Here's how the part is built. I have some questions about the finished solid (model axes, mm). Face numbers are marked on the shaded views. A direction names the side the tool comes from. Give positions to 0.01 mm unless a question says otherwise; leave off trailing zeros. Write each loop counter-clockwise with the first axis right and the second up, starting at its lowest first coordinate (ties: lowest second). Pieces come first, ordered by that corner, then holes. Notation, with made-up numbers: (23, 27.25) -> (81, 27.25) arc R11 cw to (81, 43.25) -> close; hole circle Ø1 at (86, 6.5). An arc over 180 degrees is marked (long way). Return JSON: item names as keys, results as strings.
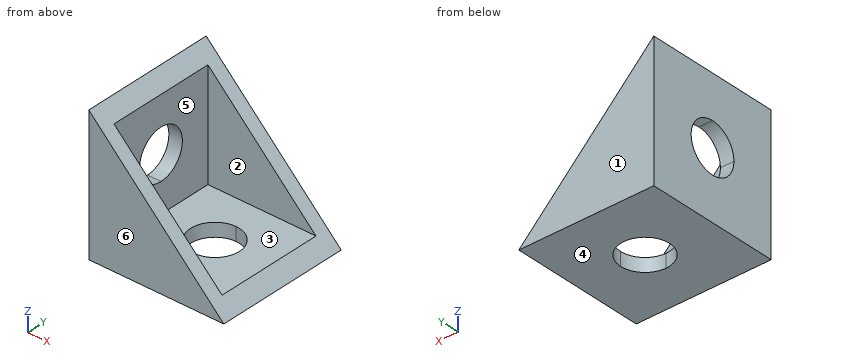
from build123d import *

# Parameters (mm, degrees)
F0_W     = 12.7
F0_H     = 12.7
F1_DEPTH = 12.7
F3_DEPTH = 25.4
F4_T     = -1.27
F7_DEPTH = 25.4
F8_DEPTH = 25.4


with BuildPart() as f1:
    # F0 (on Top) → F1 (new body)
    with BuildSketch(Plane.XY):
        with Locations((4.3248645961, 3.1129373469)):
            Rectangle(F0_W, F0_H)
    extrude(amount=F1_DEPTH)

    # F2 (on face) → F3 (cut)
    with BuildSketch(Plane.XZ.offset(3.2370626531)):
        Polygon((10.6748645961, 12.7), (-2.0251354039, 12.7), (10.6748645961, 0), align=None)
    extrude(amount=-F3_DEPTH, mode=Mode.SUBTRACT)

    # F4
    f4_openings = [f1.faces().sort_by_distance(p)[0] for p in [
        (4.324865, 3.112937, 6.35),
    ]]
    offset(amount=F4_T, openings=f4_openings)

    # F6 (on face) → F7 (cut)
    with BuildSketch(Plane(origin=(-2.0251354039, 0, 0), x_dir=(0, -1, 0), z_dir=(-1, 0, 0))):
        with BuildLine():
            ThreePointArc((-0.8015373469, 6.35), (-1.4785307329, 7.984406614), (-3.1129373469, 8.6614))
            Line((-3.1129373469, 8.6614), (-3.1129373469, 4.0386))
            ThreePointArc((-3.1129373469, 4.0386), (-1.4785307329, 4.715593386), (-0.8015373469, 6.35))
        make_face()
        with BuildLine():
            Line((-3.1129373469, 4.0386), (-3.1129373469, 8.6614))
            ThreePointArc((-3.1129373469, 8.6614), (-5.4243373469, 6.35), (-3.1129373469, 4.0386))
        make_face()
    extrude(amount=-F7_DEPTH, mode=Mode.SUBTRACT)

    # F5 (on face) → F8 (cut)
    with BuildSketch(Plane(origin=(0, 0, 0), x_dir=(1, 0, 0), z_dir=(0, 0, -1))):
        with BuildLine():
            ThreePointArc((6.6108645961, -3.1129373469), (5.9413106979, -1.4964912451), (4.3248645961, -0.8269373469))
            Line((4.3248645961, -0.8269373469), (4.3248645961, -5.3989373469))
            ThreePointArc((4.3248645961, -5.3989373469), (5.9413106979, -4.7293834487), (6.6108645961, -3.1129373469))
        make_face()
        with BuildLine():
            Line((4.3248645961, -5.3989373469), (4.3248645961, -0.8269373469))
            ThreePointArc((4.3248645961, -0.8269373469), (2.0388645961, -3.1129373469), (4.3248645961, -5.3989373469))
        make_face()
    extrude(amount=-F8_DEPTH, mode=Mode.SUBTRACT)


solid = f1.part
1. If we mould it in two halves opening along Y, with no side actions, what happens to the marked faces 3, 4, 5 and 6? For each: released by +Y, released by -Y, zero draft, split by the parting line, or undercut.
Taken from the geometry:
{"face 3": "undercut", "face 4": "zero draft", "face 5": "undercut", "face 6": "released by -Y"}
2. Suppose I cut it at A-A, the plane y = 1.75. List the corners of the cut face in (x, z) for me, and give its area (3 significant figures).
Taken from the geometry:
{"outline": "(-2.03, 0) -> (2.49, 0) -> (2.49, 1.27) -> (-0.76, 1.27) -> (-0.76, 4.48) -> (-2.03, 4.48) -> close; (-2.03, 8.22) -> (-0.76, 8.22) -> (-0.76, 11.43) -> (-2.03, 12.7) -> close; (6.16, 0) -> (10.67, 0) -> (9.4, 1.27) -> (6.16, 1.27) -> close", "area": "19.6 mm²"}
3. Suppose I cut it at C-C, the plane y = 0. List the corners of the cut face in (x, z) for me.
Taken from the geometry:
{"outline": "(-2.03, 0) -> (10.67, 0) -> (9.4, 1.27) -> (-0.76, 1.27) -> (-0.76, 11.43) -> (-2.03, 12.7) -> close"}
4. Suppose I cut it at D-D, the plane z = 9.25. List the corners of the cut face in (x, y) for me.
Taken from the geometry:
{"outline": "(-2.03, -3.24) -> (1.42, -3.24) -> (1.42, -1.97) -> (-0.76, -1.97) -> (-0.76, 8.19) -> (1.42, 8.19) -> (1.42, 9.46) -> (-2.03, 9.46) -> close"}
5. Suppose I cut it at B-B, the plane x = 2.75. List the corners of the cut face in (y, z) for me, and give its area (3 significant figures).
Taken from the geometry:
{"outline": "(-3.24, 0) -> (1.46, 0) -> (1.46, 1.27) -> (-1.97, 1.27) -> (-1.97, 7.92) -> (-3.24, 7.92) -> close; (4.77, 0) -> (9.46, 0) -> (9.46, 7.92) -> (8.19, 7.92) -> (8.19, 1.27) -> (4.77, 1.27) -> close", "area": "28.8 mm²"}
6. Which directions (+Z, -Z, +X, -X, +Y, -Y) give clear straight access to the entire face, cutting with the end or side of a thin tool? Please do the marked faces 1 and 2.
Taken from the geometry:
{"face 1": "+Z, -Z, +X, -X, +Y", "face 2": "+Z, +X"}
7. For pin 1 Ø3 at (x, y) = (6.5, 1) entering from +Z; pin 2 Ø1 at (x, z) = (6.5, 7.5) entering from -Y; pin 3 Ø5 at (y, z) = (4, 4.5) entering from +X; pin 4 Ø2 at (x, y) = (0, 5.5) entering from +Z, each with a flat end and sliding along its axis, tell me the tip position at first contact or that it passes through.
Taken from the geometry:
{"pin 1": "stops at z = 1.27", "pin 2": "passes through", "pin 3": "stops at x = -0.76", "pin 4": "stops at z = 11.67"}
8. If I drill on line 1 (Y direction, x = 2.5, z = 7.75); line 2 (Z direction, x = 7.25, y = 5.75); line 3 (X direction, y = 6.5, z = 10), over which ranges is the centre line in solid material (lowest first)? Write a range as [from, to].
Taken from the geometry:
{"line 1": "y = [-3.24, -1.97], [8.19, 9.46]", "line 2": "z = [0, 1.27]", "line 3": "x = [-2.03, -0.76]"}
